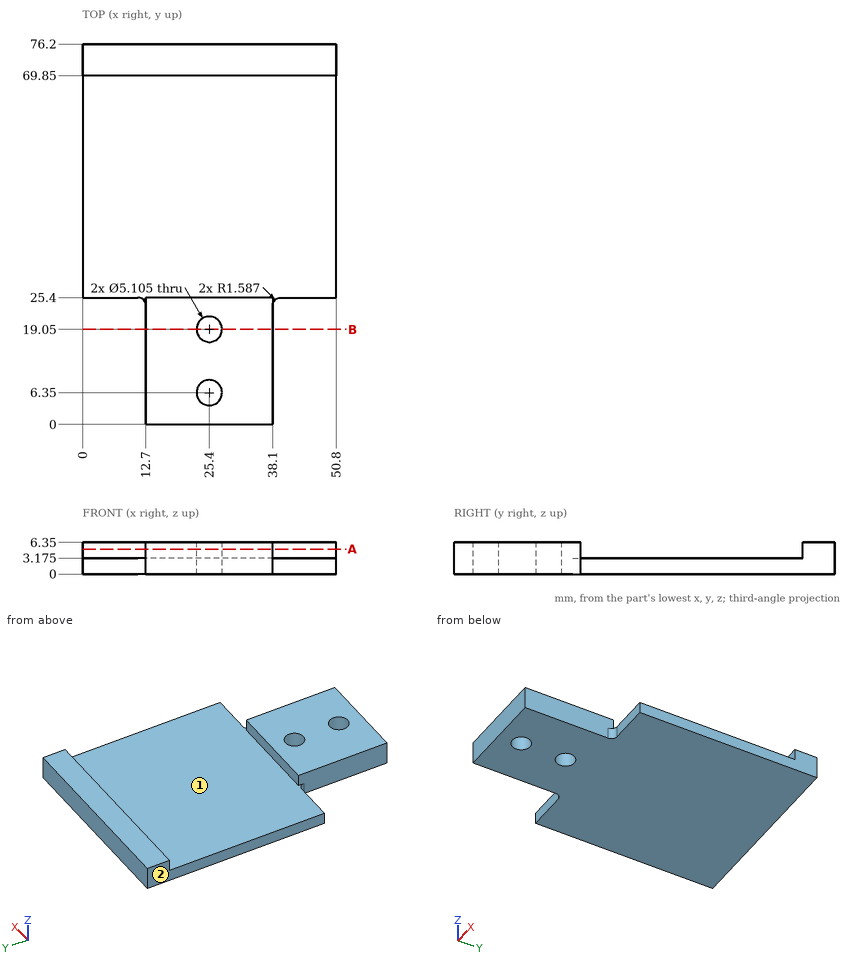
Design review of the part shown in the three views and the two pictorial views. Dimensions are in mm from the part's minimum x, y and z. Give positions to 0.01 mm unless a question says otherwise; leave off trailing zeros. Write each loop counter-clockwise with the first axis right and the second up, starting at its lowest first coordinate (ties: lowest second). Pieces come first, ordered by that corner, then holes. Notation, with made-up numbers: M 34,-8.75 L 77,-8.75 A3 cw 77,-4.75 Z; hole C 63.5,79.25 d10. An arc over 180 degrees is marked long. One line per question, with ' | ' between items. Start each with the question number.
Item 1: We need section A-A on z = 5. Give the number of separate pieces and of enclosed holes in the cut face, plus the area to 3 significant figures.
Item 2: Draft analysis for pull direction Y (two halves, no side actions). For the marked faces 1 and 2, state which applies: released by +Y, released by -Y, zero draft, split by the parting line, or undercut.
Item 3: Wall thickness on line 1 (Y direction, x = 25.4, z = 4.75); line 2 (Y direction, x = 25.4, z = 2); line 3 (X direction, y = 19.05, z = 3.25): over which ranges is each line inside the solid? List them lowest first. Write a range as from..to.
Item 4: For pin 1 (3 mm diameter, centred on y = 17, z = 4.5, fed in from +X); pin 2 (3 mm diameter, centred on x = 25.4, y = 6.35, fed in from -Z); pin 3 (1.6 mm diameter, centred on x = 8, z = 1.5, fed in from -Y), all flat-tipped, find the tip position at first contact; note any pin that passes through.
Item 5: We need section B-B on y = 19.05. Write out the cut boundary in (x, z).
Results found:
1) separate pieces: 2 | enclosed holes: 2 | area: 927 mm2
2) face 1: undercut | face 2: zero draft
3) line 1: y = 0..3.8, 8.9..16.5, 21.6..25.4, 69.85..76.2 | line 2: y = 0..3.8, 8.9..16.5, 21.6..76.2 | line 3: x = 12.7..22.85, 27.95..38.1
4) pin 1: stops at x = 38.1 | pin 2: passes through | pin 3: stops at y = 25.4
5) outline: M 12.7,0 L 22.85,0 L 22.85,6.35 L 12.7,6.35 Z; M 27.95,0 L 38.1,0 L 38.1,6.35 L 27.95,6.35 Z
